Check sheet for the modelled part. Datum: model origin and axes. Units: mm. A direction names the side the tool comes from. Give positions to 0.01 mm unless a question says otherwise; leave off trailing zeros. Write each loop counter-clockwise with the first axis right and the second up, starting at its lowest first coordinate (ties: lowest second). Pieces come first, ordered by that corner, then holes. Notation, with made-up numbers: (89, 66) -> (98, 66) arc R23 cw to (98, 85) -> close; hole circle Ø5 at (0, 56.5). An arc over 180 degrees is marked (long way). Use a Markdown table: item, result. Add a question column.
1. Cross-section at B-B (z = 13.75). Enter the section's corners in (x, y), then the cut area to 3 significant figures.
2. Set-up check for faces 4 (the flat face through (-30, -10.2, -0.2)), 5 (the flat face through (-8, -4, 0)), 6 (the flat face through (-17.4, -12.5, -15.1)): record each of +Z, -Z, +X, -X, +Y, -Y from which the full face is reachable in a straight line by a thin tool's end or side.
3. Release check for a two-part mould opening along Z. For faces 1 (the flat face through (-5, -14, -4)), 2 (the cylindrical face through (-14.524, -6.162, -12.809)), 3 (the flat face through (-12.93, -4.056, 15.243)) record: released by +Z, released by -Z, zero draft, split by the parting line, or undercut.
4. Cross-section at C-C (y = -5.25). Enter the section's corners in (x, z).
5. Gauge pin test, flat ends, axial feed: P1, Ø4, axis at x = -25, z = -13.75, coming from the -Y side; P2, Ø5, axis at x = 9, y = -8, coming from the -Z side; P3, Ø2.5, axis at x = 11.25, z = -9.59, coming from the +Y side; P4, Ø2.5, axis at y = -3, z = 3.5, coming from the +X side. Record the tip position at first contact, or that the pin passes through.
6. Scan lines: probe 1 along X at (y, z) = (-10.15, 0); probe 2 along X at (y, z) = (-9.75, 0); probe 3 along Z at (x, y) = (21, -9). Record each from-to range of solid material in increasing order. Write a range as [from, to].
7. Cross-section at D-D (x = 12). Enter the section's corners in (y, z), then the cut area to 3 significant figures.
8. Cross-section at A-A (x = -25). Enter the section's corners in (y, z).
from build123d import *
from OCP.BRepFilletAPI import BRepFilletAPI_MakeChamfer

# Parameters (mm, degrees)
BOSS_EXTRUDE1_DEPTH      = 14
BOSS_EXTRUDE1_DEPTH_BACK = 14
SKETCH1_R                = 5.1
SKETCH2_R                = 10
CUT_EXTRUDE1_DEPTH       = 20
CUT_EXTRUDE2_DEPTH       = 98
SKETCH4_R                = 2
SKETCH4_R_2              = 1.75
CUT_EXTRUDE3_DEPTH       = 98
CUT_EXTRUDE4_DEPTH       = 8
CHAMFER2_SIZE            = 10
CHAMFER2_SIZE2           = 4.452286853
SKETCH6_R                = 3.25
CUT_EXTRUDE5_DEPTH       = 1.5
SKETCH7_R                = 4.25
CUT_EXTRUDE6_DEPTH       = 1.5


with BuildPart() as part:
    # Sketch1 → Boss-Extrude1 (new, two sides: drawn at the far end of the back side and taken through both)
    # profile 1 of 7: a face of its own
    with BuildSketch(Plane(origin=(0, 0, 0), x_dir=(1, 0, 0), z_dir=(0, 1, 0)).offset(-BOSS_EXTRUDE1_DEPTH_BACK)):
        with BuildLine():
            Line((30, -6), (30, -6.397691035))
            Line((30, -6.397691035), (32.082434223, -5.627030097))
            ThreePointArc((32.082434223, -5.627030097), (31.057785286, -5.906021528), (30, -6))
        make_face()
    # profile 2 of 7: a face of its own
    with BuildSketch(Plane(origin=(0, 0, 0), x_dir=(1, 0, 0), z_dir=(0, 1, 0)).offset(-BOSS_EXTRUDE1_DEPTH_BACK)):
        with BuildLine():
            ThreePointArc((30, 6), (24, 0), (30, -6))
            Line((30, -6), (30, -2.1))
            ThreePointArc((30, -2.1), (27.9, 0), (30, 2.1))
            Line((30, 2.1), (30, 6))
        make_face()
    # profile 3 of 7: a face of its own
    with BuildSketch(Plane(origin=(0, 0, 0), x_dir=(1, 0, 0), z_dir=(0, 1, 0)).offset(-BOSS_EXTRUDE1_DEPTH_BACK)):
        with BuildLine():
            Line((30, -2.1), (30, -6))
            ThreePointArc((30, -6), (31.057785286, -5.906021528), (32.082434223, -5.627030097))
            ThreePointArc((32.082434223, -5.627030097), (34.924155021, -3.428220724), (36, 0))
            ThreePointArc((36, 0), (34.924155021, 3.428220724), (32.082434223, 5.627030097))
            ThreePointArc((32.082434223, 5.627030097), (31.057785286, 5.906021528), (30, 6))
            Line((30, 6), (30, 2.1))
            ThreePointArc((30, 2.1), (31.48492424, 1.48492424), (32.1, 0))
            ThreePointArc((32.1, 0), (31.48492424, -1.48492424), (30, -2.1))
        make_face()
    # profile 4 of 7: a face of its own
    with BuildSketch(Plane(origin=(0, 0, 0), x_dir=(1, 0, 0), z_dir=(0, 1, 0)).offset(-BOSS_EXTRUDE1_DEPTH_BACK)):
        with BuildLine():
            Line((32.082434223, 5.627030097), (30, 6.397691035))
            Line((30, 6.397691035), (30, 6))
            ThreePointArc((30, 6), (31.057785286, 5.906021528), (32.082434223, 5.627030097))
        make_face()
    # profile 5 of 7: a face of its own
    with BuildSketch(Plane(origin=(0, 0, 0), x_dir=(1, 0, 0), z_dir=(0, 1, 0)).offset(-BOSS_EXTRUDE1_DEPTH_BACK)):
        with BuildLine():
            Line((-30, 17.5), (-30, -17.5))
            Line((-30, -17.5), (0, -17.5))
            Line((0, -17.5), (30, -6.397691035))
            Line((30, -6.397691035), (30, -6))
            ThreePointArc((30, -6), (24, 0), (30, 6))
            Line((30, 6), (30, 6.397691035))
            Line((30, 6.397691035), (0, 17.5))
            Line((0, 17.5), (-30, 17.5))
        make_face()
        with Locations(Location((0, 0, 0), (0, 0, 270))):
            Circle(SKETCH1_R, mode=Mode.SUBTRACT)
    # profile 6 of 7: a face of its own
    with BuildSketch(Plane(origin=(0, 0, 0), x_dir=(1, 0, 0), z_dir=(0, 1, 0)).offset(-BOSS_EXTRUDE1_DEPTH_BACK)):
        with BuildLine():
            ThreePointArc((30, 6), (24, 0), (30, -6))
            Line((30, -6), (30, -2.1))
            ThreePointArc((30, -2.1), (27.9, 0), (30, 2.1))
            Line((30, 2.1), (30, 6))
        make_face()
    # profile 7 of 7: a face of its own
    with BuildSketch(Plane(origin=(0, 0, 0), x_dir=(1, 0, 0), z_dir=(0, 1, 0)).offset(-BOSS_EXTRUDE1_DEPTH_BACK)):
        with BuildLine():
            Line((30, -2.1), (30, -6))
            ThreePointArc((30, -6), (31.057785286, -5.906021528), (32.082434223, -5.627030097))
            ThreePointArc((32.082434223, -5.627030097), (34.924155021, -3.428220724), (36, 0))
            ThreePointArc((36, 0), (34.924155021, 3.428220724), (32.082434223, 5.627030097))
            ThreePointArc((32.082434223, 5.627030097), (31.057785286, 5.906021528), (30, 6))
            Line((30, 6), (30, 2.1))
            ThreePointArc((30, 2.1), (31.48492424, 1.48492424), (32.1, 0))
            ThreePointArc((32.1, 0), (31.48492424, -1.48492424), (30, -2.1))
        make_face()
    extrude(amount=BOSS_EXTRUDE1_DEPTH + BOSS_EXTRUDE1_DEPTH_BACK)

    # Sketch2 → Cut-Extrude1 (cut)
    with BuildSketch(Plane.ZY.offset(30)):
        Circle(SKETCH2_R)
    extrude(amount=-CUT_EXTRUDE1_DEPTH, mode=Mode.SUBTRACT)

    # Sketch3 → Cut-Extrude2 (cut)
    with BuildSketch(Plane.ZY.offset(30)):
        Polygon((-28.780571792, 0), (30.767977005, 0), (25.762660172, 25.983482973), (-26.204305774, 26.645951377), align=None)
    extrude(amount=-CUT_EXTRUDE2_DEPTH, mode=Mode.SUBTRACT)

    # Sketch4 → Cut-Extrude3 (cut)
    with BuildSketch(Plane(origin=(0, 0, 0), x_dir=(1, 0, 0), z_dir=(0, 1, 0))):
        with Locations(Location((0, 13.75, 0), (0, 0, 270))):
            Circle(SKETCH4_R)
        with Locations(Location((-25, 13.75, 0), (0, 0, 270))):
            Circle(SKETCH4_R_2)
        with Locations(Location((-16, 13.75, 0), (0, 0, 270))):
            Circle(SKETCH4_R_2)
        with Locations(Location((-16, -13.75, 0), (0, 0, 270))):
            Circle(SKETCH4_R_2)
        with Locations(Location((-25, -13.75, 0), (0, 0, 270))):
            Circle(SKETCH4_R_2)
        with Locations(Location((11.254060193, 9.585131554, 0), (0, 0, 270))):
            Circle(SKETCH4_R)
        with Locations(Location((22.508120386, 5.420263108, 0), (0, 0, 270))):
            Circle(SKETCH4_R)
        with Locations(Location((22.508120386, -5.420263108, 0), (0, 0, 270))):
            Circle(SKETCH4_R)
        with Locations(Location((11.254060193, -9.585131554, 0), (0, 0, 270))):
            Circle(SKETCH4_R)
        with Locations(Location((0, -13.75, 0), (0, 0, 270))):
            Circle(SKETCH4_R)
    extrude(amount=-CUT_EXTRUDE3_DEPTH, mode=Mode.SUBTRACT)

    # Sketch5 → Cut-Extrude4 (cut)
    with BuildSketch(Plane(origin=(0, 0, 0), x_dir=(1, 0, 0), z_dir=(0, 1, 0))):
        Polygon((-8, 24.0496753), (-8, -23.963165676), (49.955299995, -27.912565933), (56.964446833, 12.889933884), align=None)
    extrude(amount=-CUT_EXTRUDE4_DEPTH, mode=Mode.SUBTRACT)

    # Chamfer2: one chamfer whose edges measure the first distance from different faces: ONE call of the kernel's chamfer builder (chamfer() names one face for all edges)
    chamfer2_edges_1 = [part.edges().sort_by_distance(p)[0] for p in [
        (-8, -4, 17.5),
    ]]
    chamfer2_side_1 = [part.faces().sort_by_distance(p)[0] for p in [
        (-16.97752809, -7.539325843, 17.5),
    ]]
    chamfer2_edges_2 = [part.edges().sort_by_distance(p)[0] for p in [
        (-8, -4, -17.5),
    ]]
    chamfer2_side_2 = [part.faces().sort_by_distance(p)[0] for p in [
        (-16.97752809, -7.539325843, -17.5),
    ]]
    chamfer2 = BRepFilletAPI_MakeChamfer(part.part.solid().wrapped)
    for e in chamfer2_edges_1:
        chamfer2.Add(CHAMFER2_SIZE, CHAMFER2_SIZE2, e.wrapped, chamfer2_side_1[0].wrapped)  # the first distance lies on this face
    for e in chamfer2_edges_2:
        chamfer2.Add(CHAMFER2_SIZE, CHAMFER2_SIZE2, e.wrapped, chamfer2_side_2[0].wrapped)  # the first distance lies on this face
    add(Compound.cast(chamfer2.Shape()), mode=Mode.REPLACE)

    # Sketch6 → Cut-Extrude5 (cut)
    with BuildSketch(Plane.XZ.offset(14)):
        with Locations(Location((-25, 13.75, 0), (0, 0, 270))):
            Circle(SKETCH6_R)
        with Locations(Location((-16, 13.75, 0), (0, 0, 270))):
            Circle(SKETCH6_R)
        with Locations(Location((-25, -13.75, 0), (0, 0, 270))):
            Circle(SKETCH6_R)
        with Locations(Location((-16, -13.75, 0), (0, 0, 270))):
            Circle(SKETCH6_R)
    extrude(amount=-CUT_EXTRUDE5_DEPTH, mode=Mode.SUBTRACT)

    # Sketch7 → Cut-Extrude6 (cut)
    with BuildSketch(Plane.XZ.offset(14)):
        with Locations(Location((30, 0, 0), (0, 0, 270))):
            Circle(SKETCH7_R)
    extrude(amount=-CUT_EXTRUDE6_DEPTH, mode=Mode.SUBTRACT)


solid = part.part
Worked answers:
| question | item | result |
|---|---|---|
| 1 | outline | (-30, -14) -> (-28.25, -14) -> (-28.25, -12.5) -> (-26.75, -12.5) -> (-26.75, 0) -> (-30, 0) -> close; (-23.25, -12.5) -> (-21.75, -12.5) -> (-21.75, -14) -> (-19.25, -14) -> (-19.25, -12.5) -> (-17.75, -12.5) -> (-17.75, 0) -> (-23.25, 0) -> close; (-14.25, -12.5) -> (-12.75, -12.5) -> (-12.75, -14) -> (-2, -14) -> (-2, -8) -> (-9.58, -8) -> (-9.58, 0) -> (-14.25, 0) -> close; (2, -14) -> (10.13, -14) -> (10.13, -8) -> (2, -8) -> close |
| 1 | area | 273 mm² |
| 2 | face 4 | +Z, -Z, -X, +Y, -Y |
| 2 | face 5 | +Z, -Z, +X, +Y |
| 2 | face 6 | -Y |
| 3 | face 1 | zero draft |
| 3 | face 2 | undercut |
| 3 | face 3 | released by +Z |
| 4 | outline | (-30, -17.5) -> (-18, -17.5) -> (-8, -13.05) -> (-8, 13.05) -> (-18, 17.5) -> (-30, 17.5) -> (-30, 8.51) -> (-10, 8.51) -> (-10, -8.51) -> (-30, -8.51) -> close; hole circle Ø3.5 at (-25, -13.75); hole circle Ø3.5 at (-25, 13.75); hole circle Ø3.5 at (-16, -13.75); hole circle Ø3.5 at (-16, 13.75) |
| 5 | P1 | stops at y = -12.5 |
| 5 | P2 | stops at z = -15.09 |
| 5 | P3 | passes through |
| 5 | P4 | stops at x = -8 |
| 6 | probe 1 | x = [-30, -5.1], [5.1, 27.9], [32.1, 36] |
| 6 | probe 2 | x = [-10, -5.1], [5.1, 27.9], [32.1, 36] |
| 6 | probe 3 | z = [-9.73, -6.73], [-4.11, 4.11], [6.73, 9.73] |
| 7 | outline | (-14, -13.06) -> (-8, -13.06) -> (-8, -11.44) -> (-14, -11.44) -> close; (-14, -7.73) -> (-8, -7.73) -> (-8, 7.73) -> (-14, 7.73) -> close; (-14, 11.44) -> (-8, 11.44) -> (-8, 13.06) -> (-14, 13.06) -> close |
| 7 | area | 112 mm² |
| 8 | outline | (-14, -17.5) -> (0, -17.5) -> (0, -15.5) -> (-12.5, -15.5) -> (-12.5, -17) -> (-14, -17) -> close; (-14, -10.5) -> (-12.5, -10.5) -> (-12.5, -12) -> (0, -12) -> (0, -10) arc R10 cw to (0, 10) -> (0, 12) -> (-12.5, 12) -> (-12.5, 10.5) -> (-14, 10.5) -> close; (-14, 17) -> (-12.5, 17) -> (-12.5, 15.5) -> (0, 15.5) -> (0, 17.5) -> (-14, 17.5) -> close |
